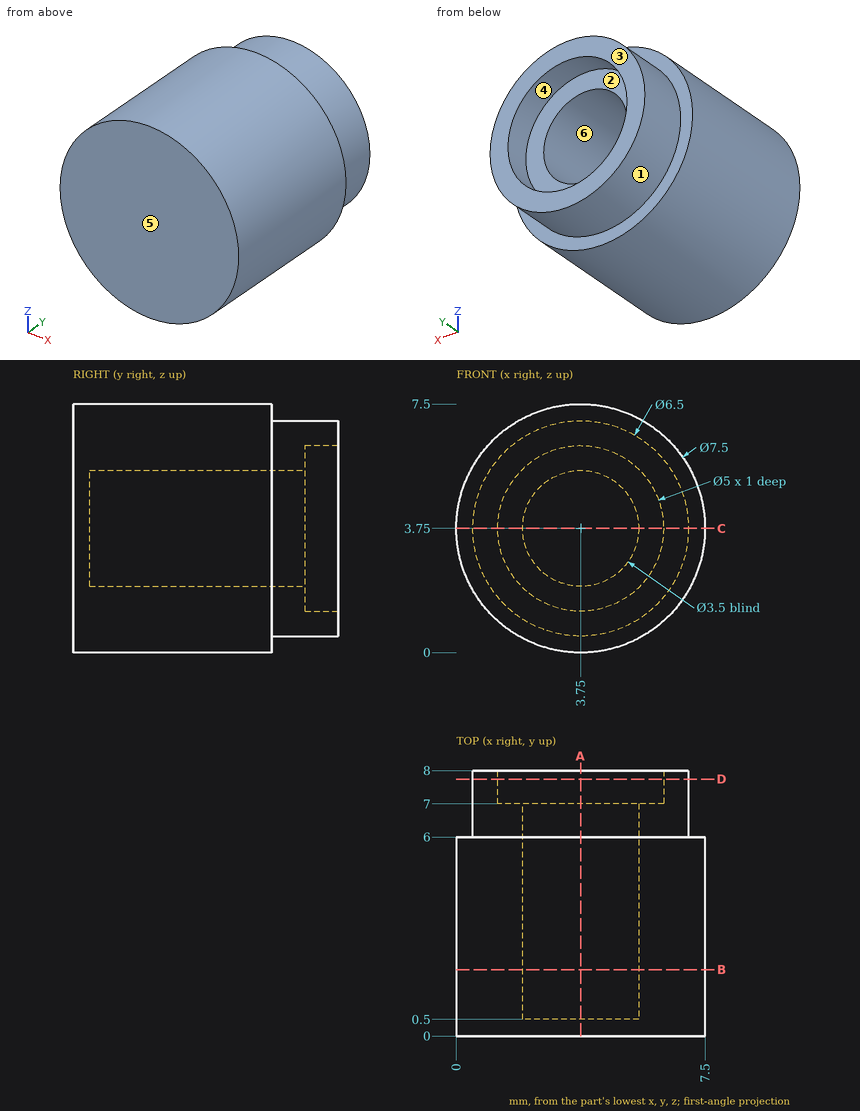
Drawing for the job (mm, zero at the part's lowest x, y, z). A direction names the side the tool comes from. Give positions to 0.01 mm unless a question says otherwise; leave off trailing zeros. Order: outer loops, then holes, each group sorted by start corner. A loop starts at its lowest first (then second) coordinate and runs counter-clockwise, first axis right, second up. Notation, with made-up numbers: M 18.25,81.5 L 49.25,81.5 A9 ccw 49.25,90.5 Z; hole C -7.5,50.5 d10. An arc over 180 degrees is marked long. Put each result on its own line as item: value. Start each with the question number.
(1) Drill centre lines: line 1 along X through (y, z) = (7.6, 3.75); line 2 along Z through (x, y) = (3.75, 3). Where is each one in solid material? Low to high.
(2) Saw through at B-B, the plane y = 2. Write the cut outline in (x, z), then the cut area to 3 significant figures.
(3) Which spindle directions (+Z, -Z, +X, -X, +Y, -Y) get a long thin tool onto all of the face, cutting with end or side? Do the marked faces 5 and 6. Say none if no direction does.
(4) Saw through at C-C, the plane z = 3.75. Write the cut outline in (x, y).
(5) Saw through at A-A, the plane x = 3.75. Write the cut outline in (y, z).
(6) Saw through at D-D, the plane y = 7.75. Write the cut outline in (x, z).
(7) Flat gauge pins, fed straight in: pin 1 Ø2 at (y, z) = (4, 5) entering from +X; pin 2 Ø3 at (x, z) = (3.75, 3.75) entering from +Y; pin 3 Ø3 at (x, z) = (4, 3.5) entering from +Y. Where does each tip first touch, or does it go through?
(8) Mould opens along X. For the marked faces 1, 2, 3 and 4 say: +X half, -X half, draft (parallel to the pull), parting line (faces both ways), or undercut.
Check result:
1. line 1: x = 0.5 to 1.25, 6.25 to 7
1. line 2: z = 0 to 2, 5.5 to 7.5
2. outline: C 3.75,3.75 d7.5; hole C 3.75,3.75 d3.5
2. area: 34.6 mm2
3. face 5: +Z, -Z, +X, -X, -Y
3. face 6: +Y
4. outline: M 0,0 L 7.5,0 L 7.5,6 L 7,6 L 7,8 L 6.25,8 L 6.25,7 L 5.5,7 L 5.5,0.5 L 2,0.5 L 2,7 L 1.25,7 L 1.25,8 L 0.5,8 L 0.5,6 L 0,6 Z
5. outline: M 0,0 L 6,0 L 6,0.5 L 8,0.5 L 8,1.25 L 7,1.25 L 7,2 L 0.5,2 L 0.5,5.5 L 7,5.5 L 7,6.25 L 8,6.25 L 8,7 L 6,7 L 6,7.5 L 0,7.5 Z
6. outline: C 3.75,3.75 d6.5; hole C 3.75,3.75 d5
7. pin 1: stops at x = 7.49
7. pin 2: stops at y = 0.5
7. pin 3: stops at y = 7
8. face 1: parting line
8. face 2: undercut
8. face 3: draft
8. face 4: undercut
